Input: part model. Units: mm. Frame: model coordinates. Face numbers are marked on the shaded views. A direction names the side the tool comes from. Round coordinates to 2 decimals unless told otherwise and drop trailing zeros. Loops run counter-clockwise (first coordinate to the right, second up) from the corner with the lowest first, then second, coordinate; pieces in that order, holes last. Notation, with made-up numbers: (18.5, 6) -> (68.5, 6) arc R18 cw to (68.5, 29) -> close; hole circle Ø1 at (77, -21). An arc over 180 degrees is marked (long way). One line per question, with ' | ' between items. Start each with the question number.
Q1. Cut plane C-C on z = 5. Return loops of the section in (x, y), and give its area (3 significant figures).
Q2. Mould query, pull axis X, two halves, no side actions, for the marked faces 6, 7 and 8. Classes: pulls with the +X half, pulls with the -X half, needs draft (parallel to the pull), parting line crosses it, or undercut.
Q3. Contact query for flat-ended pins moving along their axis: P1, Ø4, axis at y = -1.5, z = 4, coming from the -X side; P2, Ø4, axis at x = 0, y = 0, coming from the -Z side. Output: stop coordinate, or through.
Q4. Access query for the marked faces 1, 2, 3, 4 and 5. Directions: +Z, -Z, +X, -X, +Y, -Y. A direction counts if a zero-diameter tool reaches every point of the face in a straight line with its end or side. Return the directions, or none.
Q5. Cut plane D-D on x = 0. Return loops of the section in (y, z), and give its area (3 significant figures).
Q6. Material intervals for L1, parallel to Y at x = 0, z = 3.75; L2, parallel to Z at x = 3.85, y = 0; L3, parallel to Y at x = 3.4, z = 2.5, sorted ascending.
Q7. Cut plane B-B on y = 0. Return loops of the section in (x, z), and give its area (3 significant figures).
Q8. Cut plane A-A on z = 2.5. Return loops of the section in (x, y).
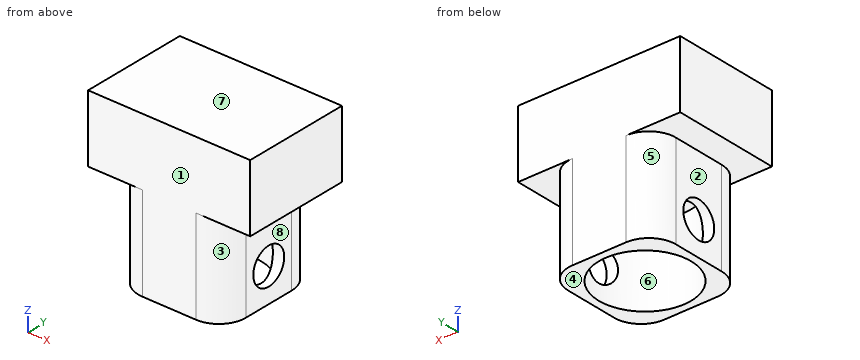
from build123d import *

# Parameters (mm, degrees)
SKETCH_1_W             = 8
SKETCH_1_H             = 8
EXTRUDE_1_DEPTH        = 7
SKETCH_1_3_OUTSIDE_W   = 12.66
SKETCH_1_3_OUTSIDE_H   = 12.66
SKETCH_1_3_OUTSIDE_W_2 = 8
SKETCH_1_3_OUTSIDE_H_2 = 8
SKETCH_1_3_OUTSIDE_R   = 3.43
CUT_EXTRUDE_1_DEPTH    = 6
SKETCH_4_R             = 1.35
CUT_EXTRUDE_2_DEPTH    = 12.6
SKETCH_8_W             = 12.06
SKETCH_8_H             = 8
EXTRUDE_3_DEPTH        = 5
FILLET_1_R             = 2


with BuildPart() as part:
    # 스케치1 → 보스-돌출1 (new body)
    with BuildSketch(Plane.XY):
        Rectangle(SKETCH_1_W, SKETCH_1_H)
    extrude(amount=EXTRUDE_1_DEPTH)

    # 스케치1<3> outside → 컷-돌출1 (cut)
    # profile 1 of 2: a face of its own
    with BuildSketch(Plane.XY):
        Rectangle(SKETCH_1_3_OUTSIDE_W, SKETCH_1_3_OUTSIDE_H)
        Rectangle(SKETCH_1_3_OUTSIDE_W_2, SKETCH_1_3_OUTSIDE_H_2, mode=Mode.SUBTRACT)
    # profile 2 of 2: a face of its own
    with BuildSketch(Plane.XY):
        Circle(SKETCH_1_3_OUTSIDE_R)
    extrude(amount=CUT_EXTRUDE_1_DEPTH, mode=Mode.SUBTRACT)

    # 스케치4 → 컷-돌출2 (cut)
    with BuildSketch(Plane(origin=(4, 0, 0), x_dir=(0, 0, -1), z_dir=(1, 0, 0))):
        with Locations((-2.5, 0)):
            Circle(SKETCH_4_R)
    extrude(amount=-CUT_EXTRUDE_2_DEPTH, mode=Mode.SUBTRACT)

    # 스케치8 → 보스-돌출3 (add)
    with BuildSketch(Plane.XY.offset(7)):
        Rectangle(SKETCH_8_W, SKETCH_8_H)
    extrude(amount=EXTRUDE_3_DEPTH)

    # 필렛1
    fillet_1_edges = [part.edges().sort_by_distance(p)[0] for p in [
        (-4, -4, 3.5),
        (4, -4, 3.5),
        (4, 4, 3.5),
        (-4, 4, 3.5),
    ]]
    fillet(fillet_1_edges, radius=FILLET_1_R)


solid = part.part
Results:
1) outline: (-4, -2) arc R2 ccw to (-2, -4) -> (2, -4) arc R2 ccw to (4, -2) -> (4, 2) arc R2 ccw to (2, 4) -> (-2, 4) arc R2 ccw to (-4, 2) -> close; hole circle Ø6.86 at (0, 0) | area: 23.6 mm^2
2) face 6: undercut | face 7: needs draft | face 8: pulls with the +X half
3) P1: x = -4 | P2: z = 6
4) face 1: +Z, -Z, +X, -X, -Y | face 2: -Z, -X, +Y, -Y | face 3: -Z, +X, -Y | face 4: -Z, +X, -X, +Y, -Y | face 5: -Z, -X, +Y
5) outline: (-4, 0) -> (-3.43, 0) -> (-3.43, 6) -> (3.43, 6) -> (3.43, 0) -> (4, 0) -> (4, 12) -> (-4, 12) -> close | area: 54.8 mm^2
6) L1: -4 to -3.43, 3.43 to 4 | L2: 0 to 1.15, 3.85 to 12 | L3: -3.43 to -1.35, 1.35 to 3.43
7) outline: (-6.03, 7) -> (-4, 7) -> (-4, 3.85) -> (-3.43, 3.85) -> (-3.43, 6) -> (3.43, 6) -> (3.43, 3.85) -> (4, 3.85) -> (4, 7) -> (6.03, 7) -> (6.03, 12) -> (-6.03, 12) -> close; (-4, 0) -> (-3.43, 0) -> (-3.43, 1.15) -> (-4, 1.15) -> close; (3.43, 0) -> (4, 0) -> (4, 1.15) -> (3.43, 1.15) -> close | area: 72.1 mm^2
8) outline: (-4, -2) arc R2 ccw to (-2, -4) -> (2, -4) arc R2 ccw to (4, -2) -> (4, -1.35) -> (3.15, -1.35) arc R3.43 cw to (-3.15, -1.35) -> (-4, -1.35) -> close; (-4, 1.35) -> (-3.15, 1.35) arc R3.43 cw to (3.15, 1.35) -> (4, 1.35) -> (4, 2) arc R2 ccw to (2, 4) -> (-2, 4) arc R2 ccw to (-4, 2) -> close
